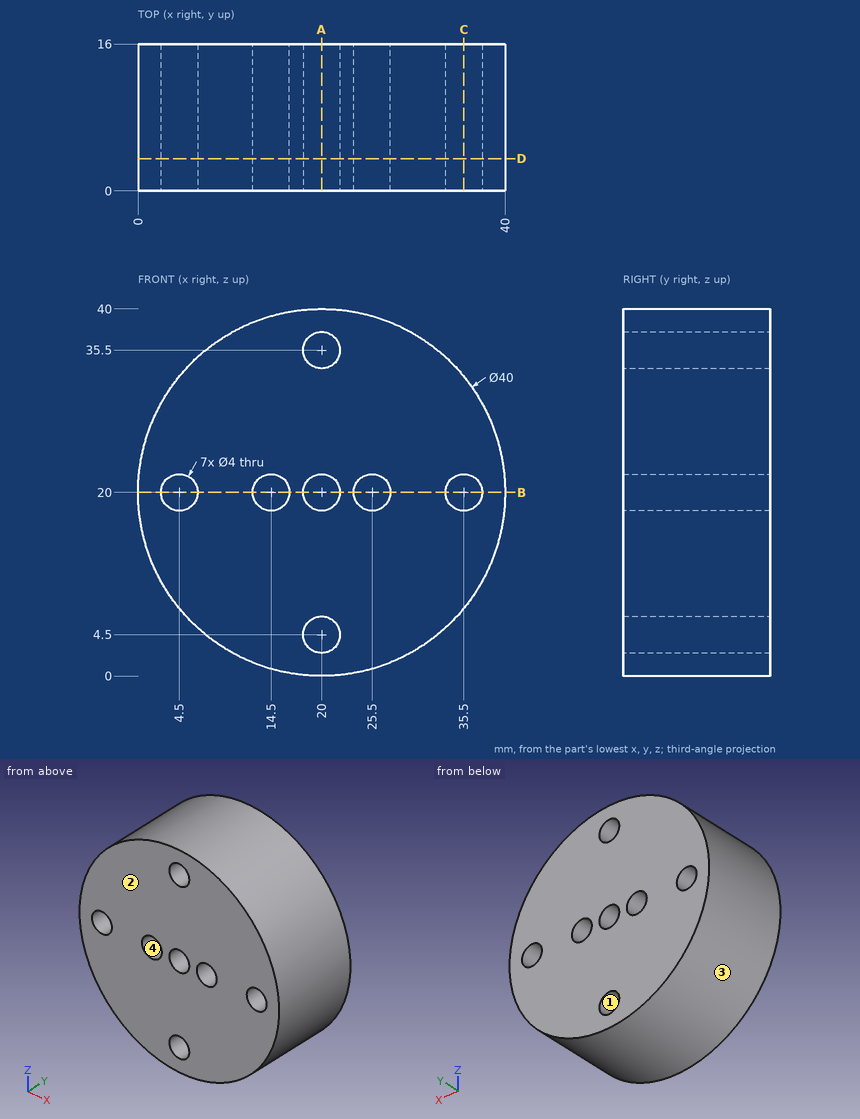
The drawing under review shows one solid part. Ordinate dimensions are in mm from its lowest x, y, z. Give positions to 0.01 mm unless a question says otherwise; leave off trailing zeros. Loops run counter-clockwise (first coordinate to the right, second up) from the corner with the lowest first, then second, coordinate; pieces in that order, holes last. Notation, with made-up numbers: M 53.5,-1.75 L 92.5,-1.75 A13 cw 92.5,7.25 Z; hole C 89,48.25 d2. An arc over 180 degrees is marked long. Return JSON: item names as keys, results as strings. Group by question number.
Item 1: Mouldability with a two-part tool opening along Z and no side actions: class the marked faces 1, 2, 3 and 4 as released by +Z, released by -Z, zero draft, split by the parting line, or undercut.
Item 2: We need section A-A (x = 20). Give the boundary of the cut face in (y, z).
Item 3: We need section B-B (z = 20). Give the boundary of the cut face in (x, y), and give its area (3 significant figures).
Item 4: We need section C-C (x = 35.5). Give the boundary of the cut face in (y, z), and give its area (3 significant figures).
Item 5: Insertion check: pin 1 Ø3 at (y, z) = (5.5, 27.5) entering from +X; pin 2 Ø2 at (x, y) = (24.5, 2) entering from +Z; pin 3 Ø2 at (x, y) = (15.5, 12) entering from -Z; pin 4 Ø4.5 at (x, z) = (14.5, 20) entering from +Y. Each pin has a flat end and moves straight along its axis. Give the tip position at first contact, or say it passes through.
Item 6: We need section D-D (y = 3.5). Give the boundary of the cut face in (x, z).
Item 7: For probe 1 along X at (y, z) = (7, 20); probe 2 along Z at (x, y) = (18.5, 5.25); probe 3 along Z at (x, y) = (19.5, 14.75), list the stretches that pass through material, from the lowest coordinate up.
Output:
{
 "1": {"face 1": "undercut", "face 2": "zero draft", "face 3": "split by the parting line", "face 4": "undercut"},
 "2": {"outline": "M 0,0 L 16,0 L 16,2.5 L 0,2.5 Z; M 0,6.5 L 16,6.5 L 16,18 L 0,18 Z; M 0,22 L 16,22 L 16,33.5 L 0,33.5 Z; M 0,37.5 L 16,37.5 L 16,40 L 0,40 Z"},
 "3": {"outline": "M 0,0 L 2.5,0 L 2.5,16 L 0,16 Z; M 6.5,0 L 12.5,0 L 12.5,16 L 6.5,16 Z; M 16.5,0 L 18,0 L 18,16 L 16.5,16 Z; M 22,0 L 23.5,0 L 23.5,16 L 22,16 Z; M 27.5,0 L 33.5,0 L 33.5,16 L 27.5,16 Z; M 37.5,0 L 40,0 L 40,16 L 37.5,16 Z", "area": "320 mm^2"},
 "4": {"outline": "M 0,7.36 L 16,7.36 L 16,18 L 0,18 Z; M 0,22 L 16,22 L 16,32.64 L 0,32.64 Z", "area": "340 mm^2"},
 "5": {"pin 1": "stops at x = 39.08", "pin 2": "stops at z = 39.69", "pin 3": "stops at z = 0.31", "pin 4": "stops at y = 16"},
 "6": {"outline": "C 20,20 d40; hole C 4.5,20 d4; hole C 14.5,20 d4; hole C 20,4.5 d4; hole C 20,20 d4; hole C 20,35.5 d4; hole C 25.5,20 d4; hole C 35.5,20 d4"},
 "7": {"probe 1": "x = 0 to 2.5, 6.5 to 12.5, 16.5 to 18, 22 to 23.5, 27.5 to 33.5, 37.5 to 40", "probe 2": "z = 0.06 to 3.18, 5.82 to 18.68, 21.32 to 34.18, 36.82 to 39.94", "probe 3": "z = 0.01 to 2.56, 6.44 to 18.06, 21.94 to 33.56, 37.44 to 39.99"}
}
